from build123d import *

# Parameters (mm, degrees)
ESQUISSE1_W             = 230
ESQUISSE1_H             = 260
BOSS_EXTRU_1_DEPTH      = 230
ESQUISSE2_W             = 222
ESQUISSE2_H             = 222
ENL_V_MAT_EXTRU_1_DEPTH = 256
ESQUISSE3_W             = 230
ESQUISSE3_H             = 230
BOSS_EXTRU_2_DEPTH      = 4
ESQUISSE4_W             = 100
ESQUISSE4_H             = 70
ENL_V_MAT_EXTRU_2_DEPTH = 456
ESQUISSE5_W             = 100
ESQUISSE5_H             = 5
BOSS_EXTRU_3_DEPTH      = 70
ESQUISSE6_W             = 100
ESQUISSE6_H             = 5
BOSS_EXTRU_4_DEPTH      = 70


with BuildPart() as part:
    # Esquisse1 → Boss.-Extru.1 (new body)
    with BuildSketch(Plane.XY):
        with Locations((115, -130)):
            Rectangle(ESQUISSE1_W, ESQUISSE1_H)
    extrude(amount=BOSS_EXTRU_1_DEPTH)

    # Esquisse2 → Enlèv. mat.-Extru.1 (cut)
    with BuildSketch(Plane.XZ.offset(260)):
        with Locations((115, 115)):
            Rectangle(ESQUISSE2_W, ESQUISSE2_H)
    extrude(amount=-ENL_V_MAT_EXTRU_1_DEPTH, mode=Mode.SUBTRACT)

    # Esquisse3 → Boss.-Extru.2 (add)
    with BuildSketch(Plane.XZ.offset(260)):
        with Locations((115, 115)):
            Rectangle(ESQUISSE3_W, ESQUISSE3_H)
    extrude(amount=-BOSS_EXTRU_2_DEPTH)

    # Esquisse4 → Enlèv. mat.-Extru.2 (cut)
    with BuildSketch(Plane.XZ.offset(260)):
        with Locations((115, 40)):
            Rectangle(ESQUISSE4_W, ESQUISSE4_H)
    extrude(amount=-ENL_V_MAT_EXTRU_2_DEPTH, mode=Mode.SUBTRACT)

    # Esquisse5 → Boss.-Extru.3 (add)
    with BuildSketch(Plane.XZ.offset(260)):
        with Locations((115, 2.5)):
            Rectangle(ESQUISSE5_W, ESQUISSE5_H)
    extrude(amount=BOSS_EXTRU_3_DEPTH)

    # Esquisse6 → Boss.-Extru.4 (add)
    with BuildSketch(Plane(origin=(0, 0, 0), x_dir=(1, 0, 0), z_dir=(0, 1, 0))):
        with Locations((115, -2.5)):
            Rectangle(ESQUISSE6_W, ESQUISSE6_H)
    extrude(amount=BOSS_EXTRU_4_DEPTH)


solid = part.part
Could you check a few things on this model? Use its own coordinates, in mm. A direction names the side the tool comes from. Coordinates: 2 decimals unless noted, no trailing zeros. Write each loop counter-clockwise with the first axis right and the second up, starting at its lowest first coordinate (ties: lowest second). Pieces come first, ordered by that corner, then holes. Notation, with made-up numbers: (69, 37) - (101, 37) arc R25 ccw to (101, 52) - close; hole circle Ø4 at (45.25, -3.75). An arc over 180 degrees is marked (long way). Write item = value, one per line.
1) Suppose I cut it at D-D on z = 98. Please give me the cut outline in (x, y).
Result set:
outline = (0, -260) - (230, -260) - (230, 0) - (0, 0) - close; hole (4, -256) - (226, -256) - (226, -4) - (4, -4) - close
2) Suppose I cut it at A-A on x = 139. Please give me the cut outline in (y, z).
Result set:
outline = (-330, 0) - (70, 0) - (70, 5) - (-4, 5) - (-4, 4) - (-256, 4) - (-256, 5) - (-330, 5) - close; (-260, 75) - (-256, 75) - (-256, 226) - (-4, 226) - (-4, 75) - (0, 75) - (0, 230) - (-260, 230) - close
3) We'd pull the mould along Y, two halves only. Please class faces 1 (the flat face through (113, -132, 4)), 2 (the flat face through (114, -292, 5)), 3 (the flat face through (113, 0, 139)): +Y half, -Y half, draft (parallel to the pull), parting line (faces both ways), or undercut.
Result set:
face_1 = undercut
face_2 = draft
face_3 = +Y half
4) For faces 4 (the flat face through (0, -132, 113)), 5 (the flat face through (4, -132, 113)), which set-ups out of +Z, -Z, +X, -X, +Y, -Y let a thin tool reach every point of the face, with its end or its side?
Result set:
face_4 = +Z, -Z, -X, +Y, -Y
face_5 = none
5) Please list where these lines run through material, in increasing order: line 1 (Z direction, x = 178, y = -40); line 2 (Y direction, x = 55, z = 33). Write a range as [from, to].
Result set:
line_1 = [0, 4], [226, 230]
line_2 = [-260, -256], [-4, 0]
6) Suppose I cut it at C-C on z = 47. Please give me the cut outline in (x, y), plus the area to 3 significant figures.
Result set:
outline = (0, -260) - (65, -260) - (65, -256) - (4, -256) - (4, -4) - (65, -4) - (65, 0) - (0, 0) - close; (165, -260) - (230, -260) - (230, 0) - (165, 0) - (165, -4) - (226, -4) - (226, -256) - (165, -256) - close
area = 3,060 mm2
7) Suppose I cut it at B-B on y = -47. Please give me the cut outline in (x, z).
Result set:
outline = (0, 0) - (230, 0) - (230, 230) - (0, 230) - close; hole (4, 4) - (226, 4) - (226, 226) - (4, 226) - close
8) Will these pins go through, and if not, where does the flat tip stop? pin 1 Ø4 at (y, z) = (35.5, 1.5) entering from +X; pin 2 Ø5.5 at (y, z) = (51, 2.5) entering from -X; pin 3 Ø4 at (x, z) = (48, 45.5) entering from -Y; pin 4 Ø1 at (x, y) = (34.5, -261) entering from +Z.
Result set:
pin_1 = 165
pin_2 = 65
pin_3 = -260
pin_4 = through
